The model under review builds one solid part; all positions refer to its coordinate system, in mm. Face numbers are marked on the shaded views. A direction names the side the tool comes from. Coordinates: 2 decimals unless noted, no trailing zeros. Write each loop counter-clockwise with the first axis right and the second up, starting at its lowest first coordinate (ties: lowest second). Pieces come first, ordered by that corner, then holes.
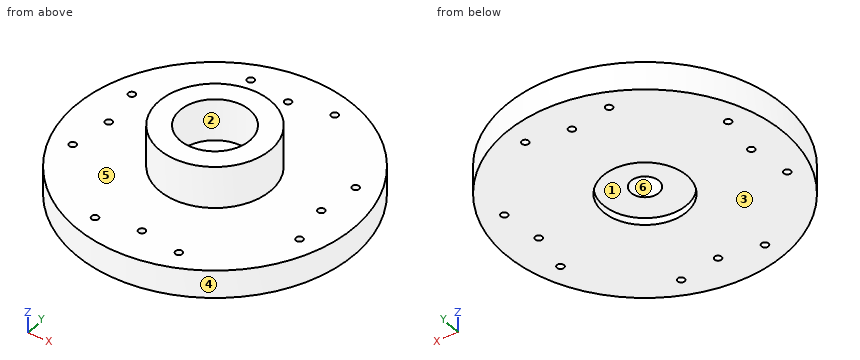
```python
from build123d import *

# Parameters (mm, degrees)
ESQUISSE1_R             = 12
ESQUISSE1_R_2           = 1.2
BOSS_EXTRU_2_DEPTH      = 2.4
ESQUISSE3_R             = 4.8
ESQUISSE3_R_2           = 3
BOSS_EXTRU_3_DEPTH      = 3.6
ESQUISSE4_R             = 0.3
ENL_V_MAT_EXTRU_1_DEPTH = 3.6
ESQUISSE5_R             = 3.6
ENL_V_MAT_EXTRU_2_DEPTH = 0.6


with BuildPart() as part:
    # Esquisse1 → Boss.-Extru.2 (new body)
    with BuildSketch(Plane.XY):
        Circle(ESQUISSE1_R)
        Circle(ESQUISSE1_R_2, mode=Mode.SUBTRACT)
    extrude(amount=BOSS_EXTRU_2_DEPTH)

    # Esquisse3 → Boss.-Extru.3 (add)
    with BuildSketch(Plane.XY.offset(2.4)):
        Circle(ESQUISSE3_R)
        Circle(ESQUISSE3_R_2, mode=Mode.SUBTRACT)
    extrude(amount=BOSS_EXTRU_3_DEPTH)

    # Esquisse4 → Enlèv. mat.-Extru.1 (cut)
    with BuildSketch(Plane.XY.offset(2.4)):
        with Locations((-9.6, -3.560674829)):
            Circle(ESQUISSE4_R)
        with Locations((-3.560674829, 9.6)):
            Circle(ESQUISSE4_R)
        with Locations((-9, 0)):
            Circle(ESQUISSE4_R)
        with Locations((-9.471169928, 3.542156917)):
            Circle(ESQUISSE4_R)
        with Locations((0, 9)):
            Circle(ESQUISSE4_R)
        with Locations((3.539325171, 9.6)):
            Circle(ESQUISSE4_R)
        with Locations((9.6, -3.560674829)):
            Circle(ESQUISSE4_R)
        with Locations((9, 0)):
            Circle(ESQUISSE4_R)
        with Locations((9.471169928, 3.542156917)):
            Circle(ESQUISSE4_R)
        with Locations((3.539325171, -9.6)):
            Circle(ESQUISSE4_R)
        with Locations((0, -9)):
            Circle(ESQUISSE4_R)
        with Locations((-3.560674829, -9.6)):
            Circle(ESQUISSE4_R)
    extrude(amount=-ENL_V_MAT_EXTRU_1_DEPTH, mode=Mode.SUBTRACT)

    # Esquisse5 → Enlèv. mat.-Extru.2 (cut)
    with BuildSketch(Plane(origin=(0, 0, 0), x_dir=(-1, 0, 0), z_dir=(0, 0, -1))):
        Circle(ESQUISSE5_R)
    extrude(amount=-ENL_V_MAT_EXTRU_2_DEPTH, mode=Mode.SUBTRACT)


solid = part.part
```
Item 1: For pin 1 (1.5 mm diameter, centred on x = -2.5, z = 4, fed in from -Y); pin 2 (3 mm diameter, centred on y = -3.5, z = 1.5, fed in from -X); pin 3 (3 mm diameter, centred on x = 0, y = 0, fed in from +Z), all flat-tipped, find the tip position at first contact; note any pin that passes through.
Solved:
pin 1: stops at y = -4.47
pin 2: stops at x = -11.83
pin 3: stops at z = 2.4
Item 2: Take a section at C-C, the plane y = -0.75. Write out the cut boundary in (x, z).
Solved:
outline: (-11.98, 0) - (-3.52, 0) - (-3.52, 0.6) - (-0.94, 0.6) - (-0.94, 2.4) - (-2.9, 2.4) - (-2.9, 6) - (-4.74, 6) - (-4.74, 2.4) - (-11.98, 2.4) - close; (0.94, 0.6) - (3.52, 0.6) - (3.52, 0) - (11.98, 0) - (11.98, 2.4) - (4.74, 2.4) - (4.74, 6) - (2.9, 6) - (2.9, 2.4) - (0.94, 2.4) - close
Item 3: Machinability: for the marked faces 1, 2 and 3, which of the approach directions +Z, -Z, +X, -X, +Y, -Y give a long, thin tool a straight path to every point of the face, cutting with its end or side? Answer none if there is none.
Solved:
face 1: -Z
face 2: +Z
face 3: -Z, +X, -X, +Y, -Y
Item 4: Take a section at B-B, the plane x = 0. Write out the cut boundary in (y, z), plus the area to 3 significant figures.
Solved:
outline: (-12, 0) - (-9.3, 0) - (-9.3, 2.4) - (-12, 2.4) - close; (-8.7, 0) - (-3.6, 0) - (-3.6, 0.6) - (-1.2, 0.6) - (-1.2, 2.4) - (-3, 2.4) - (-3, 6) - (-4.8, 6) - (-4.8, 2.4) - (-8.7, 2.4) - close; (1.2, 0.6) - (3.6, 0.6) - (3.6, 0) - (8.7, 0) - (8.7, 2.4) - (4.8, 2.4) - (4.8, 6) - (3, 6) - (3, 2.4) - (1.2, 2.4) - close; (9.3, 0) - (12, 0) - (12, 2.4) - (9.3, 2.4) - close
area: 59.0 mm2
Item 5: To check wall thickness, follow line 1 along Y through (x, z) = (0, 3.6); line 2 along Z through (x, y) = (-5.75, -7.25); line 3 along X through (y, z) = (3.75, 1.4). State the ranges of each line that lie inside material, in increasing order.
Solved:
line 1: y = -4.8 to -3, 3 to 4.8
line 2: z = 0 to 2.4
line 3: x = -11.4 to -9.69, -9.25 to 9.25, 9.69 to 11.4
Item 6: Take a section at D-D, the plane z = 4.55. Write out the cut boundary in (x, y).
Solved:
outline: circle Ø9.6 at (0, 0); hole circle Ø6 at (0, 0)
Item 7: Take a section at A-A, the plane y = 9.6. Write out the cut boundary in (x, z), plus the area to 3 significant figures.
Solved:
outline: (-7.2, 0) - (-3.86, 0) - (-3.86, 2.4) - (-7.2, 2.4) - close; (-3.26, 0) - (3.24, 0) - (3.24, 2.4) - (-3.26, 2.4) - close; (3.84, 0) - (7.2, 0) - (7.2, 2.4) - (3.84, 2.4) - close
area: 31.7 mm2
Item 8: Mouldability with a two-part tool opening along Y and no side actions: class the marked faces 4, 5 and 6 as pulls with the +Y half, pulls with the -Y half, needs draft (parallel to the pull), parting line crosses it, or undercut.
Solved:
face 4: parting line crosses it
face 5: needs draft
face 6: undercut
